Could you check a few things on this model? Use its own coordinates, in mm. Round coordinates to 2 decimals unless told otherwise and drop trailing zeros. Loops run counter-clockwise (first coordinate to the right, second up) from the corner with the lowest first, then second, coordinate; pieces in that order, holes last. Notation, with made-up numbers: (1, 42) -> (24, 42) arc R10 cw to (24, 56) -> close; hole circle Ø8 at (-14, 12.5). An arc over 180 degrees is marked (long way). Write each question's results on one line, items separated by ' | '.
from build123d import *

# Parameters (mm, degrees)
SKETCH_1_W             = 10
SKETCH_1_H             = 10
EXTRUDE_1_DEPTH        = 25
SKETCH_2_R             = 1.5
CUT_EXTRUDE_1_DEPTH    = 28.386127875
SKETCH_3_R             = 2.05
CUT_EXTRUDE_2_DEPTH    = 28.386127875
HOLE_WIZARD_M4_2_D     = 3.3
HOLE_WIZARD_M4_2_DEPTH = 10.1
HOLE_WIZARD_M4_2_TIP   = 0.991420021


with BuildPart() as part:
    # 草图1 → 凸台-拉伸1 (new body)
    with BuildSketch(Plane(origin=(0, 0, 0), x_dir=(0, 0, -1), z_dir=(1, 0, 0))):
        Rectangle(SKETCH_1_W, SKETCH_1_H)
    extrude(amount=EXTRUDE_1_DEPTH)

    # 草图2 → 切除-拉伸1 (cut, through all)
    with BuildSketch(Plane(origin=(0, 5, 0), x_dir=(1, 0, 0), z_dir=(0, 1, 0))):
        with Locations(Location((12.5, 0, 0), (0, 0, 270))):
            Circle(SKETCH_2_R)
    extrude(amount=-CUT_EXTRUDE_1_DEPTH, mode=Mode.SUBTRACT)

    # 草图3 → 切除-拉伸2 (cut, through all)
    with BuildSketch(Plane.XY.offset(5)):
        with Locations((5, 0)):
            Circle(SKETCH_3_R)
        with Locations((20, 0)):
            Circle(SKETCH_3_R)
    extrude(amount=-CUT_EXTRUDE_2_DEPTH, mode=Mode.SUBTRACT)

    # M4 螺纹孔2
    with Locations(Plane(origin=(0, 5, 0), x_dir=(1, 0, 0), z_dir=(0, 1, 0))):
        with Locations((12.5, 0)):
            Hole(HOLE_WIZARD_M4_2_D / 2, depth=HOLE_WIZARD_M4_2_DEPTH)
            with Locations((0, 0, -(HOLE_WIZARD_M4_2_DEPTH + HOLE_WIZARD_M4_2_TIP / 2))):  # 118° drill point
                Cone(0, HOLE_WIZARD_M4_2_D / 2, HOLE_WIZARD_M4_2_TIP, mode=Mode.SUBTRACT)


solid = part.part
1) I need wall thicknesses on line 1 (Y direction, x = 5, z = 2.5); line 2 (X direction, y = -1, z = -0.5); line 3 (X direction, y = 0.5, z = -3.75). Which ranges of each line are inside material? Lowest first, please.
Model answer:
line 1: y = -5 to -2.05, 2.05 to 5 | line 2: x = 0 to 3.21, 6.79 to 10.93, 14.07 to 18.21, 21.79 to 25 | line 3: x = 0 to 3.01, 6.99 to 18.01, 21.99 to 25
2) I want a section at A-A, the plane y = 0. Write out the boundary of the cut face in (x, z), plus the area to 3 significant figures.
Model answer:
outline: (0, -5) -> (2.95, -5) -> (2.95, 5) -> (0, 5) -> close; (7.05, -5) -> (17.95, -5) -> (17.95, 5) -> (7.05, 5) -> close; (22.05, -5) -> (25, -5) -> (25, 5) -> (22.05, 5) -> close; hole circle Ø3.3 at (12.5, 0) | area: 159 mm2
3) I want a section at B-B, the plane x = 20. Write out the boundary of the cut face in (y, z).
Model answer:
outline: (-5, -5) -> (-2.05, -5) -> (-2.05, 5) -> (-5, 5) -> close; (2.05, -5) -> (5, -5) -> (5, 5) -> (2.05, 5) -> close
4) I want a section at C-C, the plane z = 3.25. Write out the boundary of the cut face in (x, y).
Model answer:
outline: (0, -5) -> (25, -5) -> (25, 5) -> (0, 5) -> close; hole circle Ø4.1 at (5, 0); hole circle Ø4.1 at (20, 0)
5) I want a section at D-D, the plane z = -0.25. Write out the boundary of the cut face in (x, y).
Model answer:
outline: (0, -5) -> (10.87, -5) -> (10.87, 5) -> (0, 5) -> close; (14.13, -5) -> (25, -5) -> (25, 5) -> (14.13, 5) -> close; hole circle Ø4.1 at (5, 0); hole circle Ø4.1 at (20, 0)
6) If we mould it in two halves opening along X, with no side actions, what happens to faces 1 (the flat face through (0, 0, 0)), 2 (the flat face through (12, 0, 5)), 3 (the cylindrical face through (10.976, -0.07, 0.632)), 4 (the cylindrical face through (2.95, 0.09, 0.07))? For each: released by +X, released by -X, zero draft, split by the parting line, or undercut.
Model answer:
face 1: released by -X | face 2: zero draft | face 3: undercut | face 4: undercut
